```python
from build123d import *

# Parameters (mm, degrees)
F0_W     = 7
F0_H     = 2
F1_DEPTH = 7
F2_R     = 2
F3_DEPTH = 25
F4_R     = 3.49999


# Not quite as in the source:
# - a fillet or chamfer is up to 0.001 mm smaller than in the source, because OpenCascade refuses the exact size


with BuildPart() as f1:
    # F0 (on Top) → F1 (new body)
    with BuildSketch(Plane.XY):
        with BuildLine():
            ThreePointArc((14.8660687473, -2), (-15, 0), (14.8660687473, 2))
            Line((14.8660687473, 2), (16.7705098312, 2))
            Line((16.7705098312, 2), (16.7705098312, 5))
            Line((16.7705098312, 5), (16.0390149323, 5))
            Line((16.0390149323, 5), (16.0390149323, 7))
            ThreePointArc((16.0390149323, 7), (-17.4675765006, -1.0647869255), (16.7705098312, -5))
            Line((16.7705098312, -5), (16.7705098312, -2))
            Line((16.7705098312, -2), (14.8660687473, -2))
        make_face()
        with BuildLine():
            Line((16.7705098312, 5), (16.7705098312, 2))
            Line((16.7705098312, 2), (17.3853386507, 2))
            ThreePointArc((17.3853386507, 2), (17.1436721965, 3.5134745793), (16.7705098312, 5))
        make_face()
        with BuildLine():
            ThreePointArc((16.7705098312, 5), (17.1436721965, 3.5134745793), (17.3853386507, 2))
            Line((17.3853386507, 2), (23.7705098312, 2))
            Line((23.7705098312, 2), (23.7705098312, 5))
            Line((23.7705098312, 5), (16.7705098312, 5))
        make_face()
        with BuildLine():
            Line((23.7705098312, -2), (17.3853386507, -2))
            ThreePointArc((17.3853386507, -2), (17.1436721965, -3.5134745793), (16.7705098312, -5))
            Line((16.7705098312, -5), (23.7705098312, -5))
            Line((23.7705098312, -5), (23.7705098312, -2))
        make_face()
        with BuildLine():
            Line((17.3853386507, -2), (16.7705098312, -2))
            Line((16.7705098312, -2), (16.7705098312, -5))
            ThreePointArc((16.7705098312, -5), (17.1436721965, -3.5134745793), (17.3853386507, -2))
        make_face()
        with Locations((20.2705098312, 6)):
            Rectangle(F0_W, F0_H)
        with BuildLine():
            Line((16.0390149323, 5), (16.7705098312, 5))
            ThreePointArc((16.7705098312, 5), (16.4352130745, 6.0111372632), (16.0390149323, 7))
            Line((16.0390149323, 7), (16.0390149323, 5))
        make_face()
        with BuildLine():
            ThreePointArc((16.0390149323, 7), (16.4352130745, 6.0111372632), (16.7705098312, 5))
            Line((16.7705098312, 5), (16.7705098312, 7))
            Line((16.7705098312, 7), (16.0390149323, 7))
        make_face()
    extrude(amount=F1_DEPTH)

    # F2 (on face) → F3 (cut)
    with BuildSketch(Plane.XZ.offset(5)):
        with Locations((20.2705098312, 3.5)):
            Circle(F2_R)
    extrude(amount=-F3_DEPTH, mode=Mode.SUBTRACT)

    # F4 (radius 3.5 in the source; OpenCascade refuses exactly that, so slightly less here)
    f4_edges = [f1.edges().sort_by_distance(p)[0] for p in [
        (23.77051, -3.5, 7),
        (23.77051, 4.5, 7),
        (23.77051, -3.5, 0),
        (23.77051, 4.5, 0),
    ]]
    fillet(f4_edges, radius=F4_R)


solid = f1.part
```
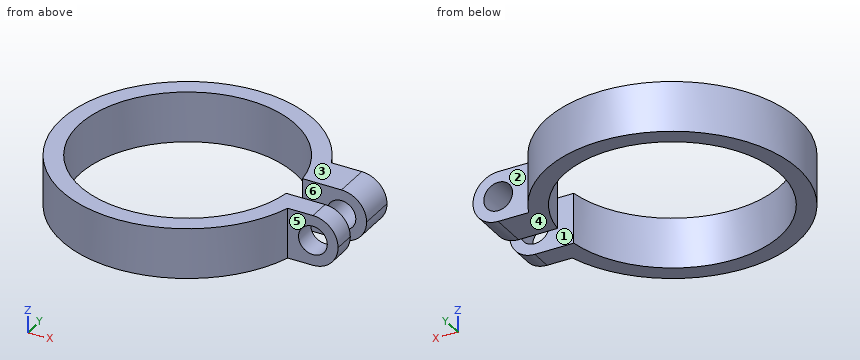
Work out the finished part from the listing and answer in its coordinate system (mm). Face numbers are marked on the shaded views. A direction names the side the tool comes from. Round coordinates to 2 decimals unless told otherwise and drop trailing zeros. Loops run counter-clockwise (first coordinate to the right, second up) from the corner with the lowest first, then second, coordinate; pieces in that order, holes last. Notation, with made-up numbers: M 13.5,5.25 L 68.5,5.25 A12 cw 68.5,18.25 Z; hole C -35,-30.5 d11. An arc over 180 degrees is marked long. One line per question, with ' | ' between items.
Q1. Find section B-B, the plane y = -11. Give the vertices of the cut face in (x, z), then the cut area to 3 significant figures.
Conclusion:
outline: M -13.61,0 L -10.2,0 L -10.2,7 L -13.61,7 Z; M 10.2,0 L 13.61,0 L 13.61,7 L 10.2,7 Z | area: 47.8 mm2
Q2. Find section D-D, the plane z = 6. Give the vertices of the cut face in (x, y).
Conclusion:
outline: M 14.87,-2 A15 cw long 14.87,2 L 22.72,2 L 22.72,7 L 16.04,7 A17.5 ccw long 16.77,-5 L 22.72,-5 L 22.72,-2 Z
Q3. Find section C-C, the plane z = 2.75. Give the vertices of the cut face in (x, y), then the cut area to 3 significant figures.
Conclusion:
outline: M 14.87,-2 A15 cw long 14.87,2 L 18.42,2 L 18.42,7 L 16.04,7 A17.5 ccw long 16.77,-5 L 18.42,-5 L 18.42,-2 Z; M 22.12,-5 L 23.69,-5 L 23.69,-2 L 22.12,-2 Z; M 22.12,2 L 23.69,2 L 23.69,7 L 22.12,7 Z | area: 269 mm2
Q4. A tool of negligible diameter and unlimited length cuts with its end or side. For the marked faces 1, 2 and 3, from which of +Z, -Z, +X, -X, +Y, -Y can it reach the whole face along a straight path? Write none if from no direction.
Conclusion:
face 1: +Z, -Z, +X | face 2: +Z, -Z, +X, +Y | face 3: +Z, +X, -X, +Y, -Y
Q5. Each of these flat-tipped pins is pushed along its axis until it touches: pin 1 Ø3.5 at (x, z) = (17.5, 4.5) entering from -Y; pin 2 Ø2 at (y, z) = (9, 1) entering from +X; pin 3 Ø2 at (x, z) = (21, 4.5) entering from +Y. Where does it stop, or does it pass through?
Conclusion:
pin 1: stops at y = -7.63 | pin 2: stops at x = 15.56 | pin 3: stops at y = 7
Q6. The mould has two halves that part along Y. Classify the marked faces 4, 5 and 6: +Y half, -Y half, draft (parallel to the pull), parting line (faces both ways), or undercut.
Conclusion:
face 4: draft | face 5: -Y half | face 6: undercut
Q7. Consider line 1 along Y through (x, z) = (18, 2.25); line 2 along Y through (x, z) = (0, 4.5); line 3 along X through (y, z) = (0, 3). Determine where each line is inside the solid, lowest interval first. Write a range as from..to.
Conclusion:
line 1: y = -5..-2, 2..7 | line 2: y = -17.5..-15, 15..17.5 | line 3: x = -17.5..-15
Q8. Find section A-A, the plane x = 0. Give the vertices of the cut face in (y, z).
Conclusion:
outline: M -17.5,0 L -15,0 L -15,7 L -17.5,7 Z; M 15,0 L 17.5,0 L 17.5,7 L 15,7 Z
